For this review, take the finished solid that the model builds, in its own axes (mm). Give positions to 0.01 mm unless a question says otherwise; leave off trailing zeros. Order: outer loops, then holes, each group sorted by start corner. A loop starts at its lowest first (then second) coordinate and runs counter-clockwise, first axis right, second up. Notation, with made-up numbers: (-15.5, 40) - (29.5, 40) arc R29 ccw to (29.5, 65) - close; hole circle Ø10 at (-28.75, -28). An arc over 180 degrees is marked (long way). Use a Markdown table: item, result. Add a question column.
1) Wall thickness on L1, parallel to Z at x = 14.5, y = 13; L2, parallel to Y at x = 11, z = -596.9 (3 decimals); L3, parallel to Z at x = 1, y = 10: over which ranges is each line inside the solid? List them lowest first.
2) We need section A-A on z = -348. Write out the cut boundary in (x, y).
3) Clearance check with flat-ended pins moving along their axes: P1, Ø4, axis at y = 12.7, z = -12.7, coming from the -X side; P2, Ø5, axis at x = 6, y = 16.5, coming from the -Z side; P3, Ø3, axis at x = 12, y = 14.5, coming from the -Z side; P4, Ø1.5, axis at x = 4, y = 18, coming from the -Z side. State where each tip first meets the part, or that it passes through.
Autodesk Inventor part; units mm, degrees
ref_plane "Work Plane1" through (0, 0, -304.8) normal (0, 0, 1) x (1, 0, 0)
ref_plane "YZ Plane" through (0, 0, 0) normal (1, 0, 0) x (0, 1, 0)
ref_plane "XZ Plane" through (0, 0, 0) normal (0, 1, 0) x (-1, 0, 0)
sketch "Sketch1" plane through (0, 0, 0) normal (1, 0, 0) x (0, 1, 0)
  line L0 (0, 0) -> (25.4, 0)
  line L1 (25.4, 0) -> (25.4, -609.6)
  line L2 (25.4, -609.6) -> (0, -609.6)
  line L3 (0, -609.6) -> (0, 0)
  dimension "d0" = 25.4
  dimension "d1" = 609.6
extrude "Extrusion1" add sketch "Sketch1" along normal blind 25.4
sketch "Sketch3" plane through (25.4, 0, 0) normal (1, 0, 0) x (0, 0, -1)
  circle A0 centre (12.7, 12.7) radius 12.7
  line L0 (609.6, 25.4) -> (0, 25.4)
  line L1 (0, 25.4) -> (0, 0)
  circle A1 centre (12.7, 12.7) radius 3.175
  dimension "d12" = 25.4
  dimension "d13" = 6.35
extrude "Extrusion3" cut sketch "Sketch3" against normal blind 25.4 contours A1
ref_plane "Work Plane1" through (0, 0, -304.8) normal (0, 0, 1) x (1, 0, 0)
mirror "Mirror1" about plane through (0, 0, -304.8) normal (0, 0, 1) of "Extrusion3"
fillet "Fillet1" radius 12.7 4 edges at (12.7, 25.4, 0) (12.7, 0, 0) (12.7, 25.4, -609.6) (12.7, 0, -609.6)
chamfer "Chamfer1" distance 2.54 angle 45 8 edges at (25.4, 25.4, -304.8) (25.4, 21.6803, -3.7197) (25.4, 0, -304.8) (25.4, 21.6803, -605.8803) (0, 25.4, -304.8) (0, 21.6803, -605.8803) (0, 0, -304.8) (0, 21.6803, -3.7197)
properties part number "bar"
Checked values:
| question | item | result |
|---|---|---|
| 1 | L1 | -609.6 to -600.06, -593.74 to -15.86, -9.54 to 0 |
| 1 | L2 | 0 to 9.525, 15.875 to 25.4 |
| 1 | L3 | -607.73 to -598.57, -595.23 to -14.37, -11.03 to -1.87 |
| 2 | outline | (0, 2.54) - (2.54, 0) - (22.86, 0) - (25.4, 2.54) - (25.4, 22.86) - (22.86, 25.4) - (2.54, 25.4) - (0, 22.86) - close |
| 3 | P1 | through |
| 3 | P2 | z = -609.53 |
| 3 | P3 | z = -609.6 |
| 3 | P4 | z = -608.76 |
